from build123d import *

# Parameters (mm, degrees)
F0_W     = 6
F0_H     = 96
F1_DEPTH = 37
F7_D     = 3
F7_DEPTH = 15
F7_TIP   = 0.9012909285
F9_D     = 3
F9_DEPTH = 15
F9_TIP   = 0.9012909285


# Not quite as in the source:
# - a feature of the source that left no trace in its solid (it failed there, or was rolled back) is left out


with BuildPart() as f1:
    # F0 (on Top) → F1 (new body)
    with BuildSketch(Plane.XY):
        with Locations((3, 48)):
            Rectangle(F0_W, F0_H)
    extrude(amount=F1_DEPTH)

    # F7
    with Locations(Plane.XZ):
        with Locations((3, 31), (3, 10)):
            Hole(F7_D / 2, depth=F7_DEPTH)
            with Locations((0, 0, -(F7_DEPTH + F7_TIP / 2))):  # 118° drill point
                Cone(0, F7_D / 2, F7_TIP, mode=Mode.SUBTRACT)

    # F9
    with Locations(Plane(origin=(0, 96, 0), x_dir=(-1, 0, 0), z_dir=(0, 1, 0))):
        with Locations((-3, 10), (-3, 31)):
            Hole(F9_D / 2, depth=F9_DEPTH)
            with Locations((0, 0, -(F9_DEPTH + F9_TIP / 2))):  # 118° drill point
                Cone(0, F9_D / 2, F9_TIP, mode=Mode.SUBTRACT)


solid = f1.part
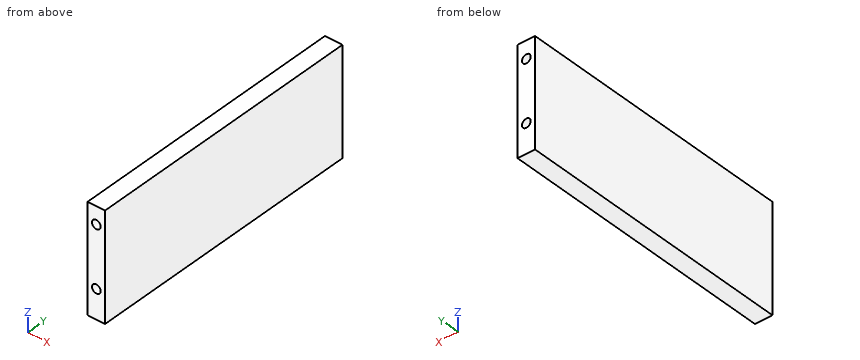
Read the model definition and answer for the solid it produces. Units are mm, in the model's axes. Round coordinates to 2 decimals unless told otherwise and drop trailing zeros. Loops run counter-clockwise (first coordinate to the right, second up) from the corner with the lowest first, then second, coordinate; pieces in that order, holes last.
Q1. Each of these flat-tipped pins is pushed along its axis until it touches: pin 1 (2.5 mm diameter, centred on x = 3, z = 10, fed in from +Y); pin 2 (2.5 mm diameter, centred on x = 3, z = 31, fed in from -Y). Where does it stop, or does it pass through?
Q2. Consider probe 1 along Z at (x, y) = (3, 11.5); probe 2 along X at (y, z) = (86.75, 31). Determine where each line is inside the solid, lowest interval first.
Q3. Section A-A on y = 90 is taken. Write down the section's boundary in (x, z), and give its area (3 significant figures).
Output:
1. pin 1: stops at y = 80.85
1. pin 2: stops at y = 15.15
2. probe 1: z = 0 to 8.5, 11.5 to 29.5, 32.5 to 37
2. probe 2: x = 0 to 1.5, 4.5 to 6
3. outline: (0, 0) - (6, 0) - (6, 37) - (0, 37) - close; hole circle Ø3 at (3, 10); hole circle Ø3 at (3, 31)
3. area: 208 mm2
